from build123d import *

# Parameters (mm, degrees)
SKETCH1_R           = 10.4
SKETCH1_R_2         = 9.5
BOSS_EXTRUDE1_DEPTH = 92.5
SKETCH3_R           = 9.5
BOSS_EXTRUDE2_DEPTH = 1.5


with BuildPart() as part:
    # Sketch1 → Boss-Extrude1 (new body)
    with BuildSketch(Plane.XY):
        Circle(SKETCH1_R)
        Circle(SKETCH1_R_2, mode=Mode.SUBTRACT)
    extrude(amount=BOSS_EXTRUDE1_DEPTH)

    # Sketch2 → Revolve1 (revolve)
    with BuildSketch(Plane(origin=(0, 0, 0), x_dir=(0, 0, -1), z_dir=(1, 0, 0)), mode=Mode.PRIVATE) as revolve1_sk:
        Polygon((0, 10.4), (1.2, 4.8), (8.2, 4.6), (8.2, 3.8), (2.2, 3.8), (2.2, 2), (10.5, 2), (10.5, 0.97), (1.2, 0.97), (1.2, 3.9), (0, 9.5), align=None)
    revolve(revolve1_sk.sketch.rotate(Axis((0, 0, 0), (0, 0, -1)), 90), axis=Axis((0, 0, 0), (0, 0, -1)))

    # Sketch3 → Boss-Extrude2 (add)
    with BuildSketch(Plane.XY.offset(92.5)):
        with BuildLine():
            Line((-3, 11.151145138), (-13.965196483, 7))
            ThreePointArc((-13.965196483, 7), (-18.8, 0), (-13.965196483, -7))
            Line((-13.965196483, -7), (-3, -11.151145138))
            ThreePointArc((-3, -11.151145138), (0, -11.7), (3, -11.151145138))
            Line((3, -11.151145138), (13.965196483, -7))
            ThreePointArc((13.965196483, -7), (18.8, 0), (13.965196483, 7))
            Line((13.965196483, 7), (3, 11.151145138))
            ThreePointArc((3, 11.151145138), (0, 11.7), (-3, 11.151145138))
        make_face()
        Circle(SKETCH3_R, mode=Mode.SUBTRACT)
    extrude(amount=BOSS_EXTRUDE2_DEPTH)


solid = part.part
The listing builds one solid part. Answer for the finished solid, in the listing's coordinates (mm). A direction names the side the tool comes from. Coordinates: 2 decimals unless noted, no trailing zeros. Loops run counter-clockwise (first coordinate to the right, second up) from the corner with the lowest first, then second, coordinate; pieces in that order, holes last. Notation, with made-up numbers: (30.25, 11) -> (36.25, 11) arc R19 cw to (36.25, 46) -> close; hole circle Ø8 at (70.25, -7.5). An arc over 180 degrees is marked (long way). Write item = value, one per line. Start each with the question number.
1) Straight lines are drawn through the part: line 1 (Y direction, x = 0, z = -6.7); line 2 (Y direction, x = 0, z = -6); line 3 (Z direction, x = -1.5, y = 10.25). For each, find the intervals that lie inside material, in ascending order. Write a range as from..to.
2) The mould has two halves that part along Y. Classify faces 1 (the face through (8.559, 9.047, 93.24)), 2 (the face through (-1, 1, -1.2)), 3 (the face through (-0.61, -4.66, -4.75)): released by +Y, released by -Y, zero draft, split by the parting line, or undercut.
3) A cutting plane is placed at C-C (z = 23). Give the vertices of the cut face in (x, y).
4) Given pin 1 Ø10 at (x, y) = (2, 7.5) entering from +Z; pin 2 Ø8 at (x, z) = (3.5, 7.5) entering from -Y; pin 3 Ø8 at (y, z) = (3.5, 19.5) entering from -X; pin 4 Ø4.5 at (x, y) = (0, 0) entering from +Z, each flat-ended and moving along its own axis, determine where each tip first touches the part or whether it passes through.
5) A tool of negligible diameter and unlimited length cuts with its end or side. For faces 4 (the face through (4.38, -8.43, 46.34)), 5 (the face through (8.406, -9.105, 93.24)), 6 (the face through (2, 2, -2.2)), from which of +Z, -Z, +X, -X, +Y, -Y can it reach the whole face along a straight path? Write none if from no direction.
6) A cutting plane is placed at D-D (x = -16). Give the vertices of the cut face in (y, z), then the cut area to 3 significant figures.
Responses:
q1.line_1 = -4.64..-3.8, -2..-0.97, 0.97..2, 3.8..4.64
q1.line_2 = -4.66..-3.8, -2..-0.97, 0.97..2, 3.8..4.66
q1.line_3 = -0.01..94
q2.face_1 = released by +Y
q2.face_2 = undercut
q2.face_3 = split by the parting line
q3.outline = circle Ø20.8 at (0, 0); hole circle Ø19 at (0, 0)
q4.pin_1 = 94
q4.pin_2 = -10.4
q4.pin_3 = -10.4
q4.pin_4 = -1.2
q5.face_4 = +Z
q5.face_5 = +Z, -Z, +X, -Y
q5.face_6 = -Z
q6.outline = (-5.84, 92.5) -> (5.84, 92.5) -> (5.84, 94) -> (-5.84, 94) -> close
q6.area = 17.5 mm²
